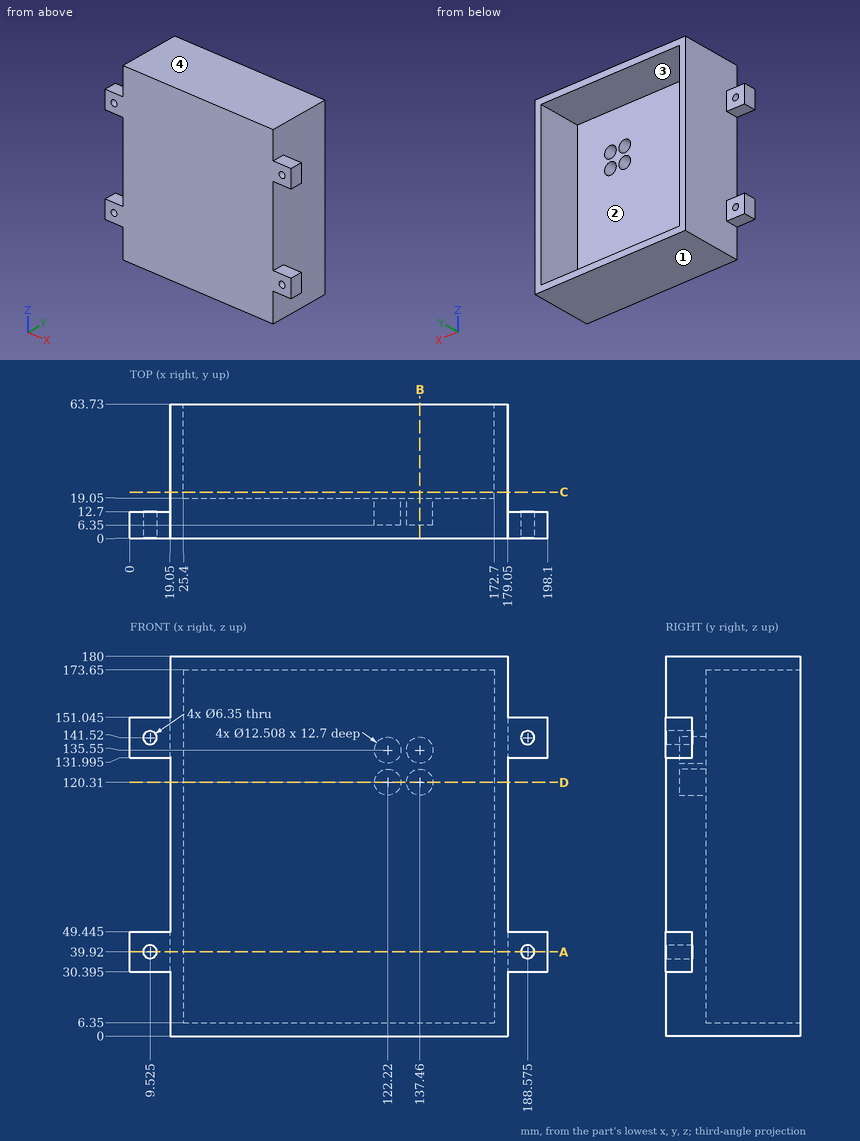
Geometry check sheet. Reference: drawing and pictorial views, mm from the part's lowest x, y, z. A direction names the side the tool comes from. Coordinates: 2 decimals unless noted, no trailing zeros. Order: outer loops, then holes, each group sorted by start corner. A loop starts at its lowest first (then second) coordinate and runs counter-clockwise, first axis right, second up. Notation, with made-up numbers: (-27.75, 84) -> (-3.75, 84) arc R8 ccw to (-3.75, 98) -> close; hole circle Ø4 at (28, -23.75). An arc over 180 degrees is marked (long way). Use CSV: the item, a comma, the result in double quotes. Start each with the question number.
Q1. Thickness scan on line 1 along X through (y, z) = (9.75, 120.31); line 2 along Z through (x, y) = (41.5, 26); line 3 along X through (y, z) = (58.5, 141). Record the ranges inside material, lowest first.
Q2. Draft check along X on the marked faces 3 and 4. Enter one of: +X half, -X half, draft (parallel to the pull), parting line (faces both ways), or undercut.
Q3. Section check B-B, the plane x = 137.46. Record the cut outline in (y, z).
Q4. Depth check by flat-ended pin: P1, Ø1, axis at x = 169.5, z = 112, coming from the +Y side; P2, Ø14, axis at x = 191, y = 3.5, coming from the -Z side (3 decimals); P3, Ø6, axis at y = 28, z = 145.5, coming from the +X side. Enter the tip coordinate at first touch or a pass-through.
Q5. Section check C-C, the plane y = 22. Record the cut outline in (x, z), and give its area (3 significant figures).
Q6. Section check A-A, the plane z = 39.92. Record the cut outline in (x, y).
Q7. Tool access check on the marked faces 1 and 2. Record the directions out of +Z, -Z, +X, -X, +Y, -Y that give a thin tool (end or side, any length) a straight path to the whole face; none if there is none.
Q8. Section check D-D, the plane z = 120.31. Record the cut outline in (x, y).
Returned:
1,line 1,"x = 19.05 to 115.97, 128.47 to 131.21, 143.71 to 179.05"
1,line 2,"z = 0 to 6.35, 173.65 to 180"
1,line 3,"x = 19.05 to 25.4, 172.7 to 179.05"
2,face 3,"undercut"
2,face 4,"draft"
3,outline,"(0, 0) -> (63.73, 0) -> (63.73, 6.35) -> (19.05, 6.35) -> (19.05, 114.06) -> (6.35, 114.06) -> (6.35, 126.56) -> (19.05, 126.56) -> (19.05, 129.3) -> (6.35, 129.3) -> (6.35, 141.8) -> (19.05, 141.8) -> (19.05, 173.65) -> (63.73, 173.65) -> (63.73, 180) -> (0, 180) -> close"
4,P1,"stops at y = 19.05"
4,P2,"stops at z = 30.395"
4,P3,"stops at x = 179.05"
5,outline,"(19.05, 0) -> (179.05, 0) -> (179.05, 180) -> (19.05, 180) -> close; hole (25.4, 6.35) -> (172.7, 6.35) -> (172.7, 173.65) -> (25.4, 173.65) -> close"
5,area,"4,160 mm^2"
6,outline,"(0, 0) -> (6.35, 0) -> (6.35, 12.7) -> (0, 12.7) -> close; (12.7, 0) -> (185.4, 0) -> (185.4, 12.7) -> (179.05, 12.7) -> (179.05, 63.73) -> (172.7, 63.73) -> (172.7, 19.05) -> (25.4, 19.05) -> (25.4, 63.73) -> (19.05, 63.73) -> (19.05, 12.7) -> (12.7, 12.7) -> close; (191.75, 0) -> (198.1, 0) -> (198.1, 12.7) -> (191.75, 12.7) -> close"
7,face 1,"-Z, +X, -X, +Y, -Y"
7,face 2,"+Y"
8,outline,"(19.05, 0) -> (179.05, 0) -> (179.05, 63.73) -> (172.7, 63.73) -> (172.7, 19.05) -> (143.71, 19.05) -> (143.71, 6.35) -> (131.21, 6.35) -> (131.21, 19.05) -> (128.47, 19.05) -> (128.47, 6.35) -> (115.97, 6.35) -> (115.97, 19.05) -> (25.4, 19.05) -> (25.4, 63.73) -> (19.05, 63.73) -> close"
